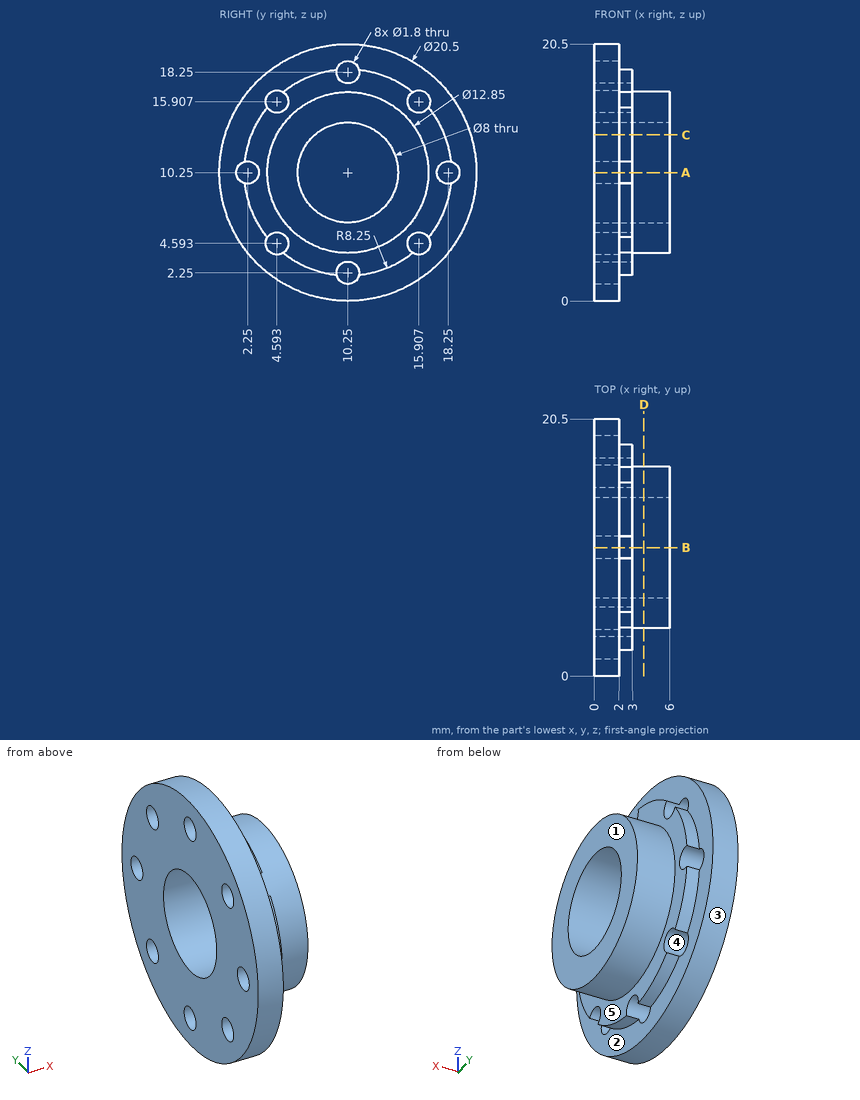
Design review of the part shown in the three views and the two pictorial views. Dimensions are in mm from the part's minimum x, y and z. A direction names the side the tool comes from. Give positions to 0.01 mm unless a question says otherwise; leave off trailing zeros. Loops run counter-clockwise (first coordinate to the right, second up) from the corner with the lowest first, then second, coordinate; pieces in that order, holes last. Notation, with made-up numbers: M -27,58.25 L -21,58.25 A19 cw -21,88.25 Z; hole C 83.5,-12.5 d11. An arc over 180 degrees is marked long. Answer as a JSON object with one key per item and string values. Group by question number.
Q1. For probe 1 along Y at (x, z) = (1.4, 10.25); probe 2 along Y at (x, z) = (5, 10.25) (3 decimals), list the stretches that pass through material, from the lowest coordinate up. Write a range as [from, to].
Q2. Add section D-D on x = 3.95. Give the boundary of the cut face in (y, z) (3 decimals), and give its area (3 significant figures).
Q3. Add section A-A on z = 10.25. Give the boundary of the cut face in (x, y) (3 decimals).
Q4. Mouldability with a two-part tool opening along Y and no side actions: class the marked faces 3, 4 and 5 as +Y half, -Y half, draft (parallel to the pull), parting line (faces both ways), or undercut.
Q5. Insertion check: P1, Ø3, axis at y = 18.25, z = 10.25, coming from the +X side; P2, Ø1.1, axis at y = 10.25, z = 18.25, coming from the +X side; P3, Ø3, axis at x = 1, z = 17.5, coming from the +Y side (1 decimal); P4, Ø1.5, axis at x = 5.5, z = 8.5, coming from the +Y side. Each pin has a flat end and moves straight along its axis. Give the tip position at first contact, or say it passes through.
Q6. Tool access review of the marked faces 1 and 2: name each direction out of +Z, -Z, +X, -X, +Y, -Y from which nothing blocks a thin tool from reaching the whole face with its end or side.
Q7. Add section C-C on z = 13.25. Give the boundary of the cut face in (x, y) (1 decimal), and give its area (3 significant figures).
Checked values:
{
 "1": {"probe 1": "[0, 1.35], [3.15, 6.25], [14.25, 17.35], [19.15, 20.5]", "probe 2": "[3.825, 6.25], [14.25, 16.675]"},
 "2": {"outline": "C 10.25,10.25 d12.85; hole C 10.25,10.25 d8", "area": "79.4 mm²"},
 "3": {"outline": "M 0,0 L 2,0 L 2,1.35 L 0,1.35 Z; M 0,3.15 L 3,3.15 L 3,3.825 L 6,3.825 L 6,6.25 L 0,6.25 Z; M 0,14.25 L 6,14.25 L 6,16.675 L 3,16.675 L 3,17.35 L 0,17.35 Z; M 0,19.15 L 2,19.15 L 2,20.5 L 0,20.5 Z"},
 "4": {"face 3": "parting line", "face 4": "undercut", "face 5": "draft"},
 "5": {"P1": "x = 3", "P2": "through", "P3": "y = 18.7", "P4": "y = 16.6"},
 "6": {"face 1": "+Z, -Z, +X, +Y, -Y", "face 2": "+X"},
 "7": {"outline": "M 0,0.4 L 2,0.4 L 2,2.6 L 3,2.6 L 3,4.6 L 6,4.6 L 6,7.6 L 0,7.6 Z; M 0,12.9 L 6,12.9 L 6,15.9 L 3,15.9 L 3,17.9 L 2,17.9 L 2,20.1 L 0,20.1 Z", "area": "56.9 mm²"}
}
